from build123d import *

# Parameters (mm, degrees)
F0_W      = 101.6
F0_H      = 101.6
F1_DEPTH  = 12.7
F2_R      = 35.56
F3_DEPTH  = 65.024
F4_W      = 101.6
F4_H      = 101.6
F4_R      = 35.56
F5_DEPTH  = 12.7
F6_R      = 5.08
F7_R      = 21.814847108
F8_DEPTH  = 101.6
F9_R      = 26.7992092516
F10_DEPTH = 5.08
F11_D     = 25.4
F11_DEPTH = 127
F11_TIP   = 7.6309298617
F12_R     = 34.29
F13_DEPTH = 91.44
F14_R     = 6.2386640532
F15_DEPTH = 12.7
F16_R     = 6.2024396885
F17_DEPTH = 12.7


with BuildPart() as f1:
    # F0 (on Top) → F1 (new body)
    with BuildSketch(Plane.XY):
        Rectangle(F0_W, F0_H)
    extrude(amount=F1_DEPTH)

    # F2 (on face) → F3 (join)
    with BuildSketch(Plane(origin=(0, 0, 0), x_dir=(1, 0, 0), z_dir=(0, 0, -1))):
        Circle(F2_R)
    extrude(amount=F3_DEPTH)

    # F4 (on face) → F5 (join)
    with BuildSketch(Plane(origin=(0, 0, -65.024), x_dir=(1, 0, 0), z_dir=(0, 0, -1))):
        Rectangle(F4_W, F4_H)
        Circle(F4_R, mode=Mode.SUBTRACT)
        Circle(F4_R)
    extrude(amount=F5_DEPTH)

    # F6
    f6_edges = [f1.edges().sort_by_distance(p)[0] for p in [
        (50.8, -50.8, 6.35),
        (-50.8, -50.8, 6.35),
        (50.8, 50.8, 6.35),
        (-50.8, 50.8, 6.35),
        (-50.8, 50.8, -71.374),
        (50.8, 50.8, -71.374),
        (50.8, -50.8, -71.374),
        (-50.8, -50.8, -71.374),
    ]]
    fillet(f6_edges, radius=F6_R)

    # F7 (on Right) → F8 (join)
    with BuildSketch(Plane.YZ):
        with Locations((0, -29.541451484)):
            Circle(F7_R)
    extrude(amount=F8_DEPTH)

    # F9 (on face) → F10 (join)
    with BuildSketch(Plane.YZ.offset(101.6)):
        with Locations((0, -29.541451484)):
            Circle(F9_R)
    extrude(amount=-F10_DEPTH)

    # F11
    with Locations(Plane.YZ.offset(101.6)):
        with Locations((0, -29.541451484)):
            Hole(F11_D / 2, depth=F11_DEPTH)
            with Locations((0, 0, -(F11_DEPTH + F11_TIP / 2))):  # 118° drill point
                Cone(0, F11_D / 2, F11_TIP, mode=Mode.SUBTRACT)

    # F12 (on face) → F13 (cut)
    with BuildSketch(Plane(origin=(0, 0, -77.724), x_dir=(1, 0, 0), z_dir=(0, 0, -1))):
        Circle(F12_R)
    extrude(amount=-F13_DEPTH, mode=Mode.SUBTRACT)

    # F14 (on face) → F15 (cut)
    with BuildSketch(Plane.XY.offset(12.7)):
        with Locations((-37.5177375972, 36.7685481906)):
            Circle(F14_R)
        with Locations((-37.5177375972, -36.7685481906)):
            Circle(F14_R)
        with Locations((37.5177375972, 36.7685481906)):
            Circle(F14_R)
        with Locations((37.5177375972, -36.7685481906)):
            Circle(F14_R)
    extrude(amount=-F15_DEPTH, mode=Mode.SUBTRACT)

    # F16 (on face) → F17 (cut)
    with BuildSketch(Plane(origin=(0, 0, -77.724), x_dir=(1, 0, 0), z_dir=(0, 0, -1))):
        with Locations((-37.392988801, 37.1180400252)):
            Circle(F16_R)
        with Locations((37.392988801, 37.1180400252)):
            Circle(F16_R)
        with Locations((-37.392988801, -37.1180400252)):
            Circle(F16_R)
        with Locations((37.392988801, -37.1180400252)):
            Circle(F16_R)
    extrude(amount=-F17_DEPTH, mode=Mode.SUBTRACT)


solid = f1.part
CAD build for the part. Positions are in the model's coordinates, mm. A direction names the side the tool comes from. Give positions to 0.01 mm unless a question says otherwise; leave off trailing zeros. Order: outer loops, then holes, each group sorted by start corner. A loop starts at its lowest first (then second) coordinate and runs counter-clockwise, first axis right, second up. Notation, with made-up numbers: (-22.5, -19.5) -> (-11.5, -19.5) arc R31 cw to (-11.5, 5.5) -> close; hole circle Ø1 at (-30, 44). An arc over 180 degrees is marked (long way). Return JSON: item names as keys, results as strings.
Q1. Saw through at D-D (z = -13.5). Write the cut outline in (x, y).
Working result:
{"outline": "(32.34, -14.78) -> (96.52, -14.78) -> (96.52, -21.47) -> (101.6, -21.47) -> (101.6, 21.47) -> (96.52, 21.47) -> (96.52, 14.78) -> (32.34, 14.78) arc R35.56 ccw (long way) to start; hole circle Ø68.58 at (0, 0)"}
Q2. Which spindle directions (+Z, -Z, +X, -X, +Y, -Y) get a long thin tool onto all of the face, cutting with end or side? Do faces 4 (the face through (-35.526, -1.564, -32.057)), 5 (the face through (32.47, 40.89, -71.46)), 6 (the face through (-34.639, -42.303, 6.439)), 7 (the face through (99.1, 25.56, -21.49)). Say none if no direction does.
Working result:
{"face 4": "none", "face 5": "-Z", "face 6": "+Z", "face 7": "+X"}
Q3. Flat gauge pins, fed straight in: pin 1 (16 mm diameter, centred on y = 11, z = -19, fed in from -X); pin 2 (12 mm diameter, centred on y = 3.5, z = -50.5, fed in from -X); pin 3 (11 mm diameter, centred on x = -37.52, y = 36.77, fed in from +Z); pin 4 (10 mm diameter, centred on y = 22.5, z = 2, fed in from +X). Where does each tip first touch, or does it go through?
Working result:
{"pin 1": "x = -35.43", "pin 2": "x = -35.56", "pin 3": "through", "pin 4": "x = 50.8"}
Q4. Mould opens along X. For faces 1 (the face through (50.8, 1, -71)), 2 (the face through (-42.315, 40.892, -71.463)), 3 (the face through (-12, -35, -65.024)) say: pulls with the +X half, pulls with the -X half, needs draft (parallel to the pull), parting line crosses it, or undercut.
Working result:
{"face 1": "pulls with the +X half", "face 2": "undercut", "face 3": "needs draft"}
Q5. Saw through at A-A (x = 0). Write the cut outline in (y, z), then the cut area to 3 significant figures.
Working result:
{"outline": "(-50.8, -77.72) -> (-34.29, -77.72) -> (-34.29, 12.7) -> (-50.8, 12.7) -> (-50.8, 0) -> (-35.56, 0) -> (-35.56, -65.02) -> (-50.8, -65.02) -> close; (34.29, -77.72) -> (50.8, -77.72) -> (50.8, -65.02) -> (35.56, -65.02) -> (35.56, 0) -> (50.8, 0) -> (50.8, 12.7) -> (34.29, 12.7) -> close", "area": "1,000 mm²"}
Q6. Drill centre lines: line 1 (Z direction, x = 36.5, y = -25); line 2 (Z direction, x = 41, y = 7.5); line 3 (X direction, y = 7, z = -14). Where is each one in solid material? Low to high.
Working result:
{"line 1": "-77.72 to -65.02, 0 to 12.7", "line 2": "-77.72 to -65.02, -50.03 to -39.79, -19.29 to -9.06, 0 to 12.7", "line 3": "-34.86 to -33.57, 33.57 to 101.6"}
Q7. Saw through at B-B (y = 0). Write the cut outline in (x, z), then the cut area to 3 significant figures.
Working result:
{"outline": "(-50.8, -77.72) -> (-34.29, -77.72) -> (-34.29, 12.7) -> (-50.8, 12.7) -> (-50.8, 0) -> (-35.56, 0) -> (-35.56, -65.02) -> (-50.8, -65.02) -> close; (34.29, -77.72) -> (50.8, -77.72) -> (50.8, -65.02) -> (35.56, -65.02) -> (35.56, -51.36) -> (96.52, -51.36) -> (96.52, -56.34) -> (101.6, -56.34) -> (101.6, -42.24) -> (34.29, -42.24) -> close; (34.29, -16.84) -> (101.6, -16.84) -> (101.6, -2.74) -> (96.52, -2.74) -> (96.52, -7.73) -> (35.56, -7.73) -> (35.56, 0) -> (50.8, 0) -> (50.8, 12.7) -> (34.29, 12.7) -> close", "area": "2,230 mm²"}
Q8. Saw through at C-C (x = 39.5). Write the cut outline in (y, z), then the cut area to 3 significant figures.
Working result:
{"outline": "(-50.8, -77.72) -> (-42.95, -77.72) -> (-42.95, -65.02) -> (-50.8, -65.02) -> close; (-50.8, 0) -> (-42.68, 0) -> (-42.68, 12.7) -> (-50.8, 12.7) -> close; (-31.28, -77.72) -> (31.28, -77.72) -> (31.28, -65.02) -> (-31.28, -65.02) -> close; (-30.85, 0) -> (30.85, 0) -> (30.85, 12.7) -> (-30.85, 12.7) -> close; circle Ø43.63 at (0, -29.54); (42.68, 0) -> (50.8, 0) -> (50.8, 12.7) -> (42.68, 12.7) -> close; (42.95, -77.72) -> (50.8, -77.72) -> (50.8, -65.02) -> (42.95, -65.02) -> close; hole circle Ø25.4 at (0, -29.54)", "area": "2,970 mm²"}
